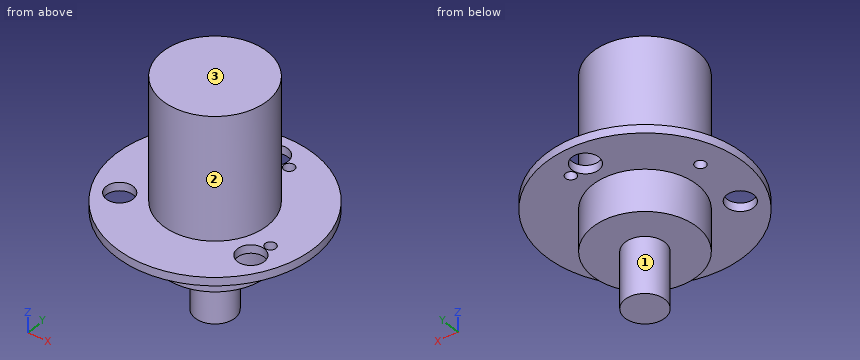
```python
from build123d import *

# Parameters (mm, degrees)
SKETCH1_R          = 6.35
EXTRUDE1_DEPTH     = 21.082
SKETCH2_R          = 2.413
EXTRUDE2_DEPTH     = 6.858
SKETCH3_R          = 12.065
EXTRUDE3_DEPTH     = 1.016
SKETCH4_R          = 1.6383
CUT_EXTRUDE1_DEPTH = 23.709219405
SKETCH6_R          = 0.65
CUT_EXTRUDE2_DEPTH = 24.392145135


with BuildPart() as part:
    # Sketch1 → Extrude1 (new body)
    with BuildSketch(Plane.XY):
        Circle(SKETCH1_R)
    extrude(amount=EXTRUDE1_DEPTH)

    # Sketch2 → Extrude2 (add)
    with BuildSketch(Plane(origin=(0, 0, 0), x_dir=(-1, 0, 0), z_dir=(0, 0, -1))):
        with Locations(Location((0, 0, 0), (0, 0, 180))):
            Circle(SKETCH2_R)
    extrude(amount=EXTRUDE2_DEPTH)

    # Sketch3 → Extrude3 (add)
    with BuildSketch(Plane(origin=(0, 0, 5.08), x_dir=(-1, 0, 0), z_dir=(0, 0, -1))):
        Circle(SKETCH3_R)
    extrude(amount=-EXTRUDE3_DEPTH)

    # Sketch4 → Cut-Extrude1 (cut, through all)
    with BuildSketch(Plane.XY.offset(6.096)):
        with Locations((0, 9.2075)):
            Circle(SKETCH4_R)
        with Locations((7.973928905, -4.60375)):
            Circle(SKETCH4_R)
        with Locations((-7.973928905, -4.60375)):
            Circle(SKETCH4_R)
    extrude(amount=-CUT_EXTRUDE1_DEPTH, mode=Mode.SUBTRACT)

    # Sketch6 → Cut-Extrude2 (cut, through all)
    with BuildSketch(Plane(origin=(0, 0, 5.08), x_dir=(-1, 0, 0), z_dir=(0, 0, -1))):
        with Locations((-8.547087459, -2.295603618)):
            Circle(SKETCH6_R)
        with Locations((-2.295603618, 8.547087459)):
            Circle(SKETCH6_R)
        with Locations((8.547087459, 2.295603618)):
            Circle(SKETCH6_R)
    extrude(amount=-CUT_EXTRUDE2_DEPTH, mode=Mode.SUBTRACT)


solid = part.part
```
Here's how the part is built. I have some questions about the finished solid (model axes, mm). Face numbers are marked on the shaded views. A direction names the side the tool comes from. Coordinates: 2 decimals unless noted, no trailing zeros. Write each loop counter-clockwise with the first axis right and the second up, starting at its lowest first coordinate (ties: lowest second). Pieces come first, ordered by that corner, then holes. Notation, with made-up numbers: M 44,83 L 64,83 A23 cw 64,107 Z; hole C 0,27.25 d1. An arc over 180 degrees is marked long. Answer as CSV lines item,"result". Start each with the question number.
Q1. Suppose I cut it at B-B, the plane y = -5.75. List the corners of the cut face in (x, z) for me, then the cut area to 3 significant figures.
Q2. Suppose I cut it at C-C, the plane x = 8.75. List the corners of the cut face in (y, z) for me.
Q3. Will these pins go through, and if not, where does the flat tip stop? pin 1 Ø6 at (x, z) = (4.5, 17) entering from +Y; pin 2 Ø5 at (x, y) = (-8.5, -4.5) entering from +Z; pin 3 Ø1.5 at (x, y) = (-8.55, 2.3) entering from -Z; pin 4 Ø10 at (y, z) = (-0.5, 5.5) entering from -X (3 decimals).
Q4. I need wall thicknesses on probe 1 along Z at (x, y) = (-6.5, 5.25); probe 2 along Z at (x, y) = (0.75, 4); probe 3 along X at (y, z) = (4, 11.5). Which ranges of each line are inside material? Lowest first, please. Write a range as [from, to].
Q5. Suppose I cut it at D-D, the plane y = 0. List the corners of the cut face in (x, z) for me (3 decimals), then the cut area to 3 significant figures.
Q6. For the marked faces 1, 2 and 3, which set-ups out of +Z, -Z, +X, -X, +Y, -Y let a thin tool reach every point of the face, with its end or its side?
Q7. Suppose I cut it at A-A, the plane x = 0. List the corners of the cut face in (y, z) for me (3 decimals).
Entries:
1,outline,"M -10.61,5.08 L -9.14,5.08 L -9.14,6.1 L -10.61,6.1 Z; M -6.8,5.08 L -2.69,5.08 L -2.69,0 L 2.69,0 L 2.69,5.08 L 6.8,5.08 L 6.8,6.1 L 2.69,6.1 L 2.69,21.08 L -2.69,21.08 L -2.69,6.1 L -6.8,6.1 Z; M 9.14,5.08 L 10.61,5.08 L 10.61,6.1 L 9.14,6.1 Z"
1,area,"125 mm²"
2,outline,"M -8.31,5.08 L -6.05,5.08 L -6.05,6.1 L -8.31,6.1 Z; M -3.16,5.08 L -2.91,5.08 L -2.91,6.1 L -3.16,6.1 Z; M -1.68,5.08 L 8.31,5.08 L 8.31,6.1 L -1.68,6.1 Z"
3,pin 1,"stops at y = 6.17"
3,pin 2,"stops at z = 6.1"
3,pin 3,"stops at z = 5.08"
3,pin 4,"stops at x = -12.065"
4,probe 1,"z = [5.08, 6.1]"
4,probe 2,"z = [0, 21.08]"
4,probe 3,"x = [-4.93, 4.93]"
5,outline,"M -12.065,5.08 L -6.35,5.08 L -6.35,0 L -2.413,0 L -2.413,-6.858 L 2.413,-6.858 L 2.413,0 L 6.35,0 L 6.35,5.08 L 12.065,5.08 L 12.065,6.096 L 6.35,6.096 L 6.35,21.082 L -6.35,21.082 L -6.35,6.096 L -12.065,6.096 Z"
5,area,"312 mm²"
6,face 1,"-Z"
6,face 2,"+Z"
6,face 3,"+Z, +X, -X, +Y, -Y"
7,outline,"M -12.065,5.08 L -6.35,5.08 L -6.35,0 L -2.413,0 L -2.413,-6.858 L 2.413,-6.858 L 2.413,0 L 6.35,0 L 6.35,5.08 L 7.569,5.08 L 7.569,6.096 L 6.35,6.096 L 6.35,21.082 L -6.35,21.082 L -6.35,6.096 L -12.065,6.096 Z; M 10.846,5.08 L 12.065,5.08 L 12.065,6.096 L 10.846,6.096 Z"
